```python
from build123d import *

# Parameters (mm, degrees)
SKETCH1_W           = 130
SKETCH1_H           = 30
SKETCH1_R           = 1.75
BOSS_EXTRUDE1_DEPTH = 4
SKETCH2_W           = 80
SKETCH2_H           = 20
CUT_EXTRUDE1_DEPTH  = 134.476589708


with BuildPart() as part:
    # Sketch1 → Boss-Extrude1 (new body)
    with BuildSketch(Plane(origin=(0, 0, 0), x_dir=(1, 0, 0), z_dir=(0, 1, 0))):
        with Locations((65, 15)):
            Rectangle(SKETCH1_W, SKETCH1_H)
        with Locations(Location((120, 25, 0), (0, 0, 270))):
            Circle(SKETCH1_R, mode=Mode.SUBTRACT)
        with Locations(Location((120, 5, 0), (0, 0, 270))):
            Circle(SKETCH1_R, mode=Mode.SUBTRACT)
        with Locations(Location((10, 5, 0), (0, 0, 270))):
            Circle(SKETCH1_R, mode=Mode.SUBTRACT)
        with Locations(Location((10, 25, 0), (0, 0, 270))):
            Circle(SKETCH1_R, mode=Mode.SUBTRACT)
    extrude(amount=BOSS_EXTRUDE1_DEPTH)

    # Sketch2 → Cut-Extrude1 (cut, through all)
    with BuildSketch(Plane(origin=(0, 4, 0), x_dir=(1, 0, 0), z_dir=(0, 1, 0))):
        with Locations((65, 15)):
            Rectangle(SKETCH2_W, SKETCH2_H)
    extrude(amount=-CUT_EXTRUDE1_DEPTH, mode=Mode.SUBTRACT)


solid = part.part
```
Geometry: final body of the model. Coordinates: model frame, mm. A direction names the side the tool comes from. Round coordinates to 2 decimals unless told otherwise and drop trailing zeros. Loops run counter-clockwise (first coordinate to the right, second up) from the corner with the lowest first, then second, coordinate; pieces in that order, holes last. Notation, with made-up numbers: (-17.75, -28) -> (26.25, -28) arc R23 ccw to (26.25, -17) -> close; hole circle Ø1 at (-21.5, -40). An arc over 180 degrees is marked (long way). Use one line per item in the form item = value. Start each with the question number.
1) Access query for faces 1 (the flat face through (64.1, 0, -25.2)), 2 (the flat face through (105, 2, -15)). Directions: +Z, -Z, +X, -X, +Y, -Y. A direction counts if a zero-diameter tool reaches every point of the face in a straight line with its end or side. Return the directions, or none.
2) Section D-D on x = 100.5. Output: boundary loops of the cut face in (y, z), then the cut area to 3 significant figures.
3) Line query: L1, parallel to Z at x = 120, y = 2.55; L2, parallel to Z at x = 64.5, y = 0.3; L3, parallel to X at y = 0.65, z = -3.75. Output: solid intervals per line, ascending.
4) Draft query along X for faces 3 (the cylindrical face through (118.29, 1.97, -5.38)), 4 (the flat face through (64, 2, 0)), 5 (the flat face through (0, 2, -15)). Return one class per face: released by +X, released by -X, zero draft, split by the parting line, or undercut.
5) First-contact query: P1, Ø3, axis at x = 120, z = -25, coming from the +Y side. Flat tip, straight axial feed; report the tip coordinate or a pass-through.
6) Section B-B on x = 10. Output: boundary loops of the cut face in (y, z).
7) Section C-C on y = 1.6. Output: boundary loops of the cut face in (x, z), then the cut area to 3 significant figures.
8) Section A-A on z = -9.25. Output: boundary loops of the cut face in (x, y).
Response:
q1.face_1 = +Z, -Z, +X, -X, -Y
q1.face_2 = +Y, -Y
q2.outline = (0, -30) -> (4, -30) -> (4, -25) -> (0, -25) -> close; (0, -5) -> (4, -5) -> (4, 0) -> (0, 0) -> close
q2.area = 40.0 mm^2
q3.L1 = -30 to -26.75, -23.25 to -6.75, -3.25 to 0
q3.L2 = -30 to -25, -5 to 0
q3.L3 = 0 to 8.78, 11.22 to 118.78, 121.22 to 130
q4.face_3 = undercut
q4.face_4 = zero draft
q4.face_5 = released by -X
q5.P1 = through
q6.outline = (0, -30) -> (4, -30) -> (4, -26.75) -> (0, -26.75) -> close; (0, -23.25) -> (4, -23.25) -> (4, -6.75) -> (0, -6.75) -> close; (0, -3.25) -> (4, -3.25) -> (4, 0) -> (0, 0) -> close
q7.outline = (0, -30) -> (130, -30) -> (130, 0) -> (0, 0) -> close; hole circle Ø3.5 at (10, -25); hole circle Ø3.5 at (10, -5); hole (25, -25) -> (105, -25) -> (105, -5) -> (25, -5) -> close; hole circle Ø3.5 at (120, -25); hole circle Ø3.5 at (120, -5)
q7.area = 2,260 mm^2
q8.outline = (0, 0) -> (25, 0) -> (25, 4) -> (0, 4) -> close; (105, 0) -> (130, 0) -> (130, 4) -> (105, 4) -> close
